from build123d import *

# Parameters (mm, degrees)
F0_R     = 1.5
F1_DEPTH = 25
F2_R     = 4
F2_R_2   = 1.5
F3_DEPTH = 0.7
F4_SIZE  = 1


with BuildPart() as f1:
    # F0 (on Top) → F1 (new body)
    with BuildSketch(Plane.XY):
        with BuildLine():
            Line((3.75, 0.4), (2.214159, 0.4))
            ThreePointArc((2.214159, 0.4), (1.59099, 1.59099), (0.4, 2.214159))
            Line((0.4, 2.214159), (0.4, 3.714159))
            Line((0.4, 3.714159), (-0.4, 3.714159))
            Line((-0.4, 3.714159), (-0.4, 2.214159))
            ThreePointArc((-0.4, 2.214159), (-1.59099, 1.59099), (-2.214159, 0.4))
            Line((-2.214159, 0.4), (-3.75, 0.4))
            Line((-3.75, 0.4), (-3.75, -0.4))
            Line((-3.75, -0.4), (-2.214159, -0.4))
            ThreePointArc((-2.214159, -0.4), (-1.59099, -1.59099), (-0.4, -2.214159))
            Line((-0.4, -2.214159), (-0.4, -3.714159))
            Line((-0.4, -3.714159), (0.4, -3.714159))
            Line((0.4, -3.714159), (0.4, -2.214159))
            ThreePointArc((0.4, -2.214159), (1.59099, -1.59099), (2.214159, -0.4))
            Line((2.214159, -0.4), (3.75, -0.4))
            Line((3.75, -0.4), (3.75, 0.4))
        make_face()
        Circle(F0_R, mode=Mode.SUBTRACT)
    extrude(amount=F1_DEPTH)

    # F2 (on face) → F3 (join)
    with BuildSketch(Plane(origin=(0, 0, 0), x_dir=(1, 0, 0), z_dir=(0, 0, -1))):
        Circle(F2_R)
        Circle(F2_R_2, mode=Mode.SUBTRACT)
    extrude(amount=F3_DEPTH)

    # F4
    f4_edges = [f1.edges().sort_by_distance(p)[0] for p in [
        (-1.5, 0, -0.7),
    ]]
    chamfer(f4_edges, length=F4_SIZE)

    # F5 (on Right) → F6 (revolve, intersect)
    with BuildSketch(Plane.YZ):
        Polygon((4.396838, 20.37701), (0, 27.094347), (0, -1.847252), (4.396838, -1.802312), align=None)
    revolve(axis=Axis((0, 0, 12.623548), (0, 0, -1)), mode=Mode.INTERSECT)


solid = f1.part
Input: part model. Units: mm. Frame: model coordinates. A direction names the side the tool comes from. Give positions to 0.01 mm unless a question says otherwise; leave off trailing zeros. Write each loop counter-clockwise with the first axis right and the second up, starting at its lowest first coordinate (ties: lowest second). Pieces come first, ordered by that corner, then holes.
Q1. Section B-B, the plane y = 0. Output: boundary loops of the cut face in (x, z).
Q2. Section D-D, the plane z = 22. Output: boundary loops of the cut face in (x, y), plus the area to 3 significant figures.
Q3. Section A-A, the plane x = 0. Output: boundary loops of the cut face in (y, z), plus the area to 3 significant figures.
Q4. Section C-C, the plane z = 2.5. Output: boundary loops of the cut face in (x, y).
Q5. First-contact query: P1, Ø1, axis at x = 1, z = 13, coming from the +Y side; P2, Ø1.2, axis at y = 3, z = 9, coming from the -X side; P3, Ø0.9, axis at y = 0, z = 7.5, coming from the +X side. Flat tips, straight axial feed; report the tip coordinate or a pass-through.
Q6. Set-up query: faces 4 (the face through (0.4, 3, 12)), 5 (the face through (1.58, -1.6, 11.66)), 6 (the face through (-1.58, 1.6, 11.66)), 7 (the face through (-1.6, -1.58, 11.66)), 8 (the face through (0, -3.714, 11)). Return all of +Z, -Z, +X, -X, +Y, -Y with unobstructed straight access to the full face (end or side cutting, diameter ignored); none if empty.
Q7. Pull-direction query (X, two-part tool) for faces 1 (the face through (-0.4, -3, 12)), 2 (the face through (1.6, 1.58, 11.66)), 3 (the face through (-1.5, -0.07, 12.72)); classes: pulls with the +X half, pulls with the -X half, needs draft (parallel to the pull), parting line crosses it, or undercut.
Q8. Material intervals for probe 1 along X at (y, z) = (0, 19); probe 2 along Y at (x, z) = (0, 17.5); probe 3 along Z at (x, y) = (-1.75, -2), sorted ascending.
Filled in:
1. outline: (-4, -0.7) - (-2.5, -0.7) - (-1.5, 0.3) - (-1.5, 24.8) - (-3.75, 21.37) - (-3.75, 0) - (-4, 0) - close; (1.5, 0.3) - (2.5, -0.7) - (4, -0.7) - (4, 0) - (3.75, 0) - (3.75, 21.37) - (1.5, 24.8) - close
2. outline: (-3.31, -0.4) - (-2.21, -0.4) arc R2.25 ccw to (-0.4, -2.21) - (-0.4, -3.31) arc R3.33 ccw to (0.4, -3.31) - (0.4, -2.21) arc R2.25 ccw to (2.21, -0.4) - (3.31, -0.4) arc R3.33 ccw to (3.31, 0.4) - (2.21, 0.4) arc R2.25 ccw to (0.4, 2.21) - (0.4, 3.31) arc R3.33 ccw to (-0.4, 3.31) - (-0.4, 2.21) arc R2.25 ccw to (-2.21, 0.4) - (-3.31, 0.4) arc R3.33 ccw to start; hole circle Ø3 at (0, 0)
2. area: 12.3 mm2
3. outline: (-4, -0.7) - (-2.5, -0.7) - (-1.5, 0.3) - (-1.5, 24.8) - (-3.71, 21.42) - (-3.71, 0) - (-4, 0) - close; (1.5, 0.3) - (2.5, -0.7) - (4, -0.7) - (4, 0) - (3.71, 0) - (3.71, 21.42) - (1.5, 24.8) - close
3. area: 105 mm2
4. outline: (-3.75, -0.4) - (-2.21, -0.4) arc R2.25 ccw to (-0.4, -2.21) - (-0.4, -3.71) - (0.4, -3.71) - (0.4, -2.21) arc R2.25 ccw to (2.21, -0.4) - (3.75, -0.4) - (3.75, 0.4) - (2.21, 0.4) arc R2.25 ccw to (0.4, 2.21) - (0.4, 3.71) - (-0.4, 3.71) - (-0.4, 2.21) arc R2.25 ccw to (-2.21, 0.4) - (-3.75, 0.4) - close; hole circle Ø3 at (0, 0)
5. P1: stops at y = 2.19
5. P2: stops at x = -0.4
5. P3: stops at x = 3.75
6. face 4: +Z, +X, +Y
6. face 5: +Z, +X, -Y
6. face 6: +Z, -X, +Y
6. face 7: +Z, -X, -Y
6. face 8: +Z, +X, -X, -Y
7. face 1: pulls with the -X half
7. face 2: pulls with the +X half
7. face 3: undercut
8. probe 1: x = -3.75 to -1.5, 1.5 to 3.75
8. probe 2: y = -3.71 to -1.5, 1.5 to 3.71
8. probe 3: z = -0.7 to 0
